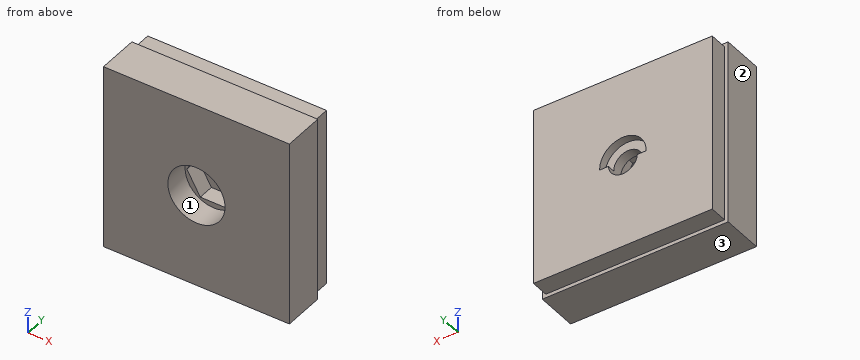
```python
from build123d import *

# Parameters (mm, degrees)
SKETCH1_W           = 52
SKETCH1_H           = 52
BOSS_EXTRUDE1_DEPTH = 11.5
SKETCH2_W           = 50
SKETCH2_H           = 50
SKETCH2_R           = 4.05
BOSS_EXTRUDE2_DEPTH = 5
SKETCH3_R           = 8
CUT_EXTRUDE1_DEPTH  = 7
CUT_EXTRUDE2_DEPTH  = 2.2


with BuildPart() as part:
    # Sketch1 → Boss-Extrude1 (new body)
    with BuildSketch(Plane(origin=(0, 0, 0), x_dir=(1, 0, 0), z_dir=(0, 1, 0))):
        with Locations((-26, 26)):
            Rectangle(SKETCH1_W, SKETCH1_H)
        Polygon((-18.494446501, 26), (-22.24722325, 32.5), (-29.75277675, 32.5), (-33.505553499, 26), (-29.75277675, 19.5), (-22.24722325, 19.5), align=None, mode=Mode.SUBTRACT)
    extrude(amount=BOSS_EXTRUDE1_DEPTH)

    # Sketch2 → Boss-Extrude2 (add)
    with BuildSketch(Plane(origin=(0, 11.5, 0), x_dir=(1, 0, 0), z_dir=(0, 1, 0))):
        with Locations((-26, 26)):
            Rectangle(SKETCH2_W, SKETCH2_H)
        with Locations(Location((-26, 26, 0), (0, 0, 270))):
            Circle(SKETCH2_R, mode=Mode.SUBTRACT)
    extrude(amount=BOSS_EXTRUDE2_DEPTH)

    # Sketch3 → Cut-Extrude1 (cut)
    with BuildSketch(Plane.XZ):
        with Locations(Location((-26, -26, 0), (0, 0, 270))):
            Circle(SKETCH3_R)
    extrude(amount=-CUT_EXTRUDE1_DEPTH, mode=Mode.SUBTRACT)

    # Sketch4 → Cut-Extrude2 (cut)
    with BuildSketch(Plane(origin=(0, 16.5, 0), x_dir=(1, 0, 0), z_dir=(0, 1, 0))):
        with BuildLine():
            Line((-32.496922348, 26.2), (-19.503077652, 26.2))
            ThreePointArc((-19.503077652, 26.2), (-26, 19.5), (-32.496922348, 26.2))
        make_face()
    extrude(amount=-CUT_EXTRUDE2_DEPTH, mode=Mode.SUBTRACT)


solid = part.part
```
Design review of the part built by this model. Coordinates are the model's own, in mm. Face numbers are marked on the shaded views. Give positions to 0.01 mm unless a question says otherwise; leave off trailing zeros. Order: outer loops, then holes, each group sorted by start corner. A loop starts at its lowest first (then second) coordinate and runs counter-clockwise, first axis right, second up. Notation, with made-up numbers: M 24,-0.75 L 49,-0.75 A33 ccw 49,34.25 Z; hole C 9.5,87 d5. An arc over 180 degrees is marked long. One line per question, with ' | ' between items. Start each with the question number.
Q1. For L1, parallel to X at y = 13.1, z = -26; L2, parallel to X at y = 15, z = -26; L3, parallel to Z at x = -39.5, y = 13.25, list the stretches that pass through material, from the lowest coordinate up. Write a range as [from, to].
Q2. The part is to be moulded in two halves that separate along Z. For the marked faces 1, 2 and 3, say which applies: +Z half, -Z half, draft (parallel to the pull), parting line (faces both ways), or undercut.
Q3. We need section B-B (y = 9.25). Write out the cut boundary in (x, z), plus the area to 3 significant figures.
Q4. We need section A-A (x = -26). Write out the cut boundary in (y, z), plus the area to 3 significant figures.
Q5. For pin 1 Ø6.5 at (x, z) = (-23.5, -24.5) entering from -Y; pin 2 Ø0.7 at (x, y) = (-31, 16) entering from +Z; pin 3 Ø4 at (x, y) = (-18, 14.5) entering from -Z, all flat-tipped, find the tip position at first contact; note any pin that passes through.
Q6. We need section C-C (z = -27). Write out the cut boundary in (x, y).
Q7. We need section D-D (y = 1.5). Write out the cut boundary in (x, z).
Returned:
1) L1: [-51, -30.05], [-21.95, -1] | L2: [-51, -32.5], [-19.5, -1] | L3: [-51, -1]
2) face 1: undercut | face 2: draft | face 3: -Z half
3) outline: M -52,-52 L 0,-52 L 0,0 L -52,0 Z; hole M -33.51,-26 L -29.75,-32.5 L -22.25,-32.5 L -18.49,-26 L -22.25,-19.5 L -29.75,-19.5 Z | area: 2,560 mm2
4) outline: M 0,-52 L 11.5,-52 L 11.5,-51 L 16.5,-51 L 16.5,-30.05 L 11.5,-30.05 L 11.5,-32.5 L 7,-32.5 L 7,-34 L 0,-34 Z; M 0,-18 L 7,-18 L 7,-19.5 L 11.5,-19.5 L 11.5,-21.95 L 14.3,-21.95 L 14.3,-19.5 L 16.5,-19.5 L 16.5,-1 L 11.5,-1 L 11.5,0 L 0,0 Z | area: 632 mm2
5) pin 1: y = 11.5 | pin 2: z = -1 | pin 3: z = -51
6) outline: M -52,0 L -33.94,0 L -33.94,7 L -32.93,7 L -32.93,11.5 L -29.92,11.5 L -29.92,16.5 L -51,16.5 L -51,11.5 L -52,11.5 Z; M -22.08,11.5 L -19.07,11.5 L -19.07,7 L -18.06,7 L -18.06,0 L 0,0 L 0,11.5 L -1,11.5 L -1,16.5 L -22.08,16.5 Z
7) outline: M -52,-52 L 0,-52 L 0,0 L -52,0 Z; hole C -26,-26 d16
